Read the model definition and answer for the solid it produces. Units are mm, in the model's axes. Face numbers are marked on the shaded views. A direction names the side the tool comes from. Round coordinates to 2 decimals unless told otherwise and drop trailing zeros. Write each loop counter-clockwise with the first axis right and the second up, starting at its lowest first coordinate (ties: lowest second). Pieces come first, ordered by that corner, then holes. Notation, with made-up numbers: (-12, -5) -> (-3, -5) arc R23 cw to (-3, 15) -> close; hole circle Ø11 at (-27, 54.25). An arc over 180 degrees is marked (long way). Return JSON: item names as keys, results as strings. Group by question number.
(1) Given pin 1 (1.5 mm diameter, centred on x = 3.5, y = 9.5, fed in from +Z); pin 2 (2 mm diameter, centred on y = 9, z = 2, fed in from -X); pin 3 (2.5 mm diameter, centred on x = 10.26, y = 7.74, fed in from -Z); pin 4 (4.5 mm diameter, centred on x = -2, z = 3, fed in from -Y), each flat-ended and moving along its own axis, determine where each tip first touches the part or whether it passes through.
(2) The mould has two halves that part along X. Classify the marked faces 4, 5, 6 and 7: released by +X, released by -X, zero draft, split by the parting line, or undercut.
(3) A cutting plane is placed at C-C on x = -13. Give the vertices of the cut face in (y, z).
(4) A cutting plane is placed at D-D on z = 0.75. Give the vertices of the cut face in (x, y) (3 decimals).
(5) Straight lines are drawn through the part: line 1 (X direction, y = 6.5, z = 4.5); line 2 (X direction, y = 6.75, z = 3.75); line 3 (Z direction, x = -5, y = 6.5). For each, find the intervals that lie inside material, in ascending order.
(6) A cutting plane is placed at B-B on z = 4.5. Give the vertices of the cut face in (x, y) (3 decimals).
(7) For the marked faces 1, 2 and 3, determine the directions among +Z, -Z, +X, -X, +Y, -Y from which every point of the face is accessible in a straight line to the end or side of a thin tool.
(8) A cutting plane is placed at A-A on z = 6.5. Give the vertices of the cut face in (x, y) (3 decimals).
```python
from build123d import *

# Parameters (mm, degrees)
F1_DEPTH = 7.62
F3_DEPTH = 4.572
F4_R     = 0.762
F5_R     = 1.905
F6_DEPTH = 7.621
F8_DEPTH = 31.751


with BuildPart() as f1:
    # F0 (on Top) → F1 (new body)
    with BuildSketch(Plane.XY):
        with BuildLine():
            ThreePointArc((-6.35, 2.54), (-5.6060512242, 4.3360512242), (-3.81, 5.08))
            Line((-3.81, 5.08), (3.81, 5.08))
            ThreePointArc((3.81, 5.08), (5.6060512242, 4.3360512242), (6.35, 2.54))
            Line((6.35, 2.54), (6.35, 1.27))
            Line((6.35, 1.27), (15.875, 1.27))
            Line((15.875, 1.27), (15.875, 5.08))
            ThreePointArc((15.875, 5.08), (13.6431536726, 10.4681536726), (8.255, 12.7))
            Line((8.255, 12.7), (-8.255, 12.7))
            ThreePointArc((-8.255, 12.7), (-13.6431536726, 10.4681536726), (-15.875, 5.08))
            Line((-15.875, 5.08), (-15.875, 1.27))
            Line((-15.875, 1.27), (-6.35, 1.27))
            Line((-6.35, 1.27), (-6.35, 2.54))
        make_face()
    extrude(amount=F1_DEPTH)

    # F2 (on face) → F3 (cut)
    with BuildSketch(Plane.XY.offset(7.62)):
        Polygon((2.153245525, 13.6789603775), (0.3542888121, 5.0024012453), (2.1943775111, 4.5093509644), (4.9747148636, 12.9229499468), align=None)
    extrude(amount=-F3_DEPTH, mode=Mode.SUBTRACT)

    # F4
    f4_edges = [f1.edges().sort_by_distance(p)[0] for p in [
        (1.160325, 8.89, 3.048),
        (3.641996, 8.89, 3.048),
    ]]
    fillet(f4_edges, radius=F4_R)

    # F5 (on face) → F6 (cut, through all)
    with BuildSketch(Plane.XY.offset(7.62)):
        with Locations((10.2573568001, 7.736901287)):
            Circle(F5_R)
    extrude(amount=-F6_DEPTH, mode=Mode.SUBTRACT)

    # F7 (on face) → F8 (cut, through all)
    with BuildSketch(Plane(origin=(-15.875, 0, 0), x_dir=(0, -1, 0), z_dir=(-1, 0, 0))):
        with BuildLine():
            Line((-3.302, 7.62), (-12.7, 7.62))
            Line((-12.7, 7.62), (-12.7, 5.588))
            Line((-12.7, 5.588), (-5.08, 5.588))
            ThreePointArc((-5.08, 5.588), (-3.8227641431, 6.1087641431), (-3.302, 7.366))
            Line((-3.302, 7.366), (-3.302, 7.62))
        make_face()
    extrude(amount=-F8_DEPTH, mode=Mode.SUBTRACT)


solid = f1.part
```
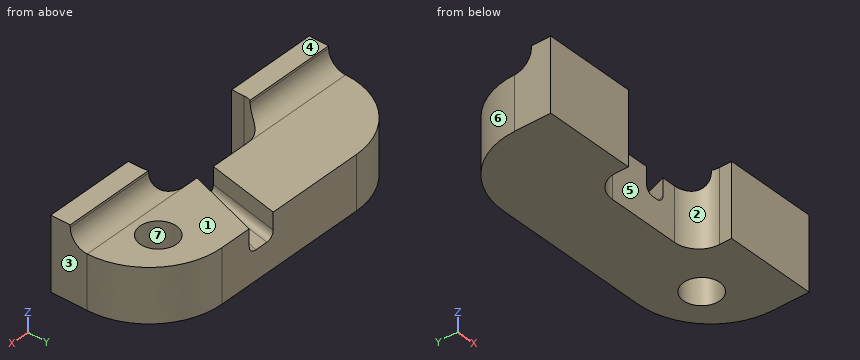
Checks:
{
 "1": {"pin 1": "stops at z = 5.59", "pin 2": "stops at x = -15.29", "pin 3": "passes through", "pin 4": "stops at y = 5.04"},
 "2": {"face 4": "zero draft", "face 5": "undercut", "face 6": "released by -X", "face 7": "undercut"},
 "3": {"outline": "(1.27, 0) -> (11.04, 0) -> (11.04, 5.59) -> (5.08, 5.59) arc R1.78 cw to (3.3, 7.37) -> (3.3, 7.62) -> (1.27, 7.62) -> close"},
 "4": {"outline": "(-15.875, 1.27) -> (-6.35, 1.27) -> (-6.35, 2.54) arc R2.54 cw to (-3.81, 5.08) -> (3.81, 5.08) arc R2.54 cw to (6.35, 2.54) -> (6.35, 1.27) -> (15.875, 1.27) -> (15.875, 5.08) arc R7.62 ccw to (8.255, 12.7) -> (-8.255, 12.7) arc R7.62 ccw to (-15.875, 5.08) -> close; hole circle Ø3.81 at (10.257, 7.737)"},
 "5": {"line 1": "x = -15.74 to 0.66, 2.85 to 8.81, 11.71 to 15.74", "line 2": "x = -15.69 to 0.72, 2.93 to 8.63, 11.89 to 15.69", "line 3": "z = 0 to 5.59"},
 "6": {"outline": "(-15.875, 1.27) -> (-6.35, 1.27) -> (-6.35, 2.54) arc R2.54 cw to (-3.81, 5.08) -> (0.37, 5.08) -> (1.95, 12.7) -> (-8.255, 12.7) arc R7.62 ccw to (-15.875, 5.08) -> close; (2.383, 5.08) -> (3.81, 5.08) arc R2.54 cw to (6.35, 2.54) -> (6.35, 1.27) -> (15.875, 1.27) -> (15.875, 5.08) arc R7.62 ccw to (8.255, 12.7) -> (4.901, 12.7) -> close; hole circle Ø3.81 at (10.257, 7.737)"},
 "7": {"face 1": "+Z, +X, -X, +Y", "face 2": "+Z, -Z, -Y", "face 3": "+Z, -Z, +X, +Y, -Y"},
 "8": {"outline": "(-15.875, 1.27) -> (-6.35, 1.27) -> (-6.35, 2.54) arc R2.54 cw to (-6.15, 3.527) -> (-15.875, 3.527) -> close; (6.15, 3.527) arc R2.54 cw to (6.35, 2.54) -> (6.35, 1.27) -> (15.875, 1.27) -> (15.875, 3.527) -> close"}
}
